```python
from build123d import *

# Parameters (mm, degrees)
BOSS_EXTRUDE1_DEPTH     = 55
CUT_EXTRUDE2_DEPTH      = 206.91260282
CUT_EXTRUDE2_DEPTH_BACK = 206.91260282
SKETCH2_W               = 100.4
SKETCH2_H               = 20.4
CUT_EXTRUDE3_DEPTH      = 20
FILLET1_R               = 45
CUT_EXTRUDE4_DEPTH      = 206.91260282
CUT_EXTRUDE4_DEPTH_BACK = 206.91260282
BOSS_EXTRUDE2_DEPTH     = 55
SKETCH29_R              = 1.75
SKETCH29_R_2            = 13
CUT_EXTRUDE5_DEPTH      = 10
SKETCH33_R              = 2.3
CUT_EXTRUDE9_DEPTH      = 10
SKETCH34_R              = 2.3
CUT_EXTRUDE10_DEPTH     = 10
FILLET2_R               = 5
CUT_EXTRUDE6_DEPTH      = 5
FILLET3_START           = 72
FILLET3_DEPTH           = 42
FILLET3_START_2         = 73.456949031
FILLET3_2_DEPTH         = 10
FILLET3_START_3         = 108.456949031
FILLET3_3_DEPTH         = 5
SKETCH31_R              = 2.3
CUT_EXTRUDE7_DEPTH      = 10
SKETCH32_R              = 2.3
CUT_EXTRUDE8_DEPTH      = 10
SKETCH35_R              = 2.3
CUT_EXTRUDE11_DEPTH     = 157.645539016
SKETCH36_R              = 4
CUT_EXTRUDE12_DEPTH     = 161.275509096
SKETCH37_R              = 2.1
CUT_EXTRUDE13_DEPTH     = 15
SKETCH38_R              = 2.3
CUT_EXTRUDE14_DEPTH     = 202.494416813
SKETCH39_R              = 4
CUT_EXTRUDE15_DEPTH     = 31
CHAMFER1_SIZE           = 1


with BuildPart() as part:
    # Sketch1 → Boss-Extrude1 (new body)
    with BuildSketch(Plane(origin=(0, 0, 0), x_dir=(1, 0, 0), z_dir=(0, 1, 0))):
        Polygon((0, 0), (150, 0), (75, 129.903810568), align=None)
    extrude(amount=-BOSS_EXTRUDE1_DEPTH)

    # Sketch4 → Cut-Extrude2 (cut, two sides: drawn at the far end of the back side and taken through both)
    with BuildSketch(Plane(origin=(0, 0, 0), x_dir=(1, 0, 0), z_dir=(0, 1, 0)).offset(-CUT_EXTRUDE2_DEPTH_BACK)):
        Polygon((58.511973189, 45.566570047), (40.845863577, 35.365169595), (51.047264029, 17.699059984), (68.713373641, 27.900460435), align=None)
    extrude(amount=CUT_EXTRUDE2_DEPTH + CUT_EXTRUDE2_DEPTH_BACK, mode=Mode.SUBTRACT)

    # Sketch2 → Cut-Extrude3 (cut)
    with BuildSketch(Plane(origin=(0, 0, 0), x_dir=(1, 0, 0), z_dir=(0, 1, 0))):
        Polygon((109.197045256, 138.33483042), (58.997045256, 51.38587988), (41.330127019, 61.58587988), (91.530127019, 148.53483042), align=None)
        with Locations((124.2, 15.2)):
            Rectangle(SKETCH2_W, SKETCH2_H)
    extrude(amount=-CUT_EXTRUDE3_DEPTH, mode=Mode.SUBTRACT)

    # Fillet1
    fillet1_edges = [part.edges().sort_by_distance(p)[0] for p in [
        (0, -27.5, 0),
    ]]
    fillet(fillet1_edges, radius=FILLET1_R)

    # Sketch27 → Cut-Extrude4 (cut, two sides: drawn at the far end of the back side and taken through both)
    with BuildSketch(Plane(origin=(0, 0, 0), x_dir=(1, 0, 0), z_dir=(0, 1, 0)).offset(-CUT_EXTRUDE4_DEPTH_BACK)):
        Polygon((238.272822489, 351.900634614), (92.551448183, 99.503810568), (65.734741667, 53.05591239), (78.81753352, 30.4), (132.448551817, 30.4), (423.891300428, 30.4), (928.68494852, 321.842748611), (743.066470581, 643.343383225), align=None)
    extrude(amount=CUT_EXTRUDE4_DEPTH + CUT_EXTRUDE4_DEPTH_BACK, mode=Mode.SUBTRACT)

    # Sketch28 → Boss-Extrude2 (add)
    with BuildSketch(Plane(origin=(0, 0, 0), x_dir=(1, 0, 0), z_dir=(0, 1, 0))):
        Polygon((83.054457118, 83.054539524), (113.460135283, 30.4), (107.686368323, 30.4), (80.167837876, 78.054768335), align=None)
    extrude(amount=-BOSS_EXTRUDE2_DEPTH)

    # Sketch29 → Cut-Extrude5 (cut)
    with BuildSketch(Plane(origin=(98.252102834, 0, -56.73626329), x_dir=(-0.5000686496051991, 0, -0.8659857652883405), z_dir=(0.8659857652883404, 0, -0.500068649605199))):
        with Locations((-15.510385308, -12)):
            Circle(SKETCH29_R)
        with Locations((15.489614692, -12)):
            Circle(SKETCH29_R)
        with Locations((15.489614692, -43)):
            Circle(SKETCH29_R)
        with Locations((-15.510385308, -43)):
            Circle(SKETCH29_R)
        with Locations((-0.010385308, -27.5)):
            Circle(SKETCH29_R_2)
    extrude(amount=-CUT_EXTRUDE5_DEPTH, mode=Mode.SUBTRACT)

    # Sketch33 → Cut-Extrude9 (cut)
    with BuildSketch(Plane(origin=(26.327172275, 0, 15.2), x_dir=(0.4999999999999997, 0, -0.8660254037844388), z_dir=(0.8660254037844389, 0, 0.49999999999999983))):
        with Locations((122.448551817, -10)):
            Circle(SKETCH33_R)
    extrude(amount=-CUT_EXTRUDE9_DEPTH, mode=Mode.SUBTRACT)

    # Sketch34 → Cut-Extrude10 (cut)
    with BuildSketch(Plane(origin=(0, 0, -30.4), x_dir=(-1, 0, 0), z_dir=(0, 0, -1))):
        with Locations((-122.448551817, -10)):
            Circle(SKETCH34_R)
    extrude(amount=-CUT_EXTRUDE10_DEPTH, mode=Mode.SUBTRACT)

    # Fillet2
    fillet2_edges = [part.edges().sort_by_distance(p)[0] for p in [
        (107.686368323, -27.5, -30.4),
        (113.460135283, -27.5, -30.4),
        (83.054457118, -27.5, -83.054539524),
        (80.167837876, -27.5, -78.054768335),
        (65.734741667, -27.5, -53.05591239),
        (78.81753352, -27.5, -30.4),
    ]]
    fillet(fillet2_edges, radius=FILLET2_R)

    # Sketch30 → Cut-Extrude6 (cut)
    with BuildSketch(Plane.XZ.offset(55)):
        Polygon((62.116998953, -39.323625207), (122.736002524, -74.32843068), (125.736414421, -69.132516088), (65.117410851, -34.127710616), align=None)
    extrude(amount=-CUT_EXTRUDE6_DEPTH, mode=Mode.SUBTRACT)

    # Fillet3: read off the stored shape, not the designer's step
    # Fillet3 outline → Fillet3 (cut)
    with BuildSketch(Plane(origin=(0, 0, 0), x_dir=(0.5000686496051991, 0, 0.8659857652883406), z_dir=(0.8659857652883404, 0, -0.5000686496051993)).offset(FILLET3_START)):
        with BuildLine():
            Line((-2.990935885, 55), (-5.490935885, 55))
            ThreePointArc((-5.490935885, 55), (-3.723168932, 54.267766953), (-2.990935885, 52.5))
            Line((-2.990935885, 52.5), (-2.990935885, 55))
        make_face()
        with BuildLine():
            Line((5.509064115, 55), (3.009064115, 55))
            Line((3.009064115, 55), (3.009064115, 52.5))
            ThreePointArc((3.009064115, 52.5), (3.741297162, 54.267766953), (5.509064115, 55))
        make_face()
    extrude(amount=FILLET3_DEPTH, mode=Mode.SUBTRACT)

    # Fillet3 2 outline → Fillet3 2 (add)
    with BuildSketch(Plane(origin=(0, 0, 0), x_dir=(0.5000686496051991, 0, 0.8659857652883406), z_dir=(0.8659857652883404, 0, -0.5000686496051993)).offset(FILLET3_START_2)):
        with BuildLine():
            ThreePointArc((-0.490935885, 50), (-2.258702838, 50.732233047), (-2.990935885, 52.5))
            Line((-2.990935885, 52.5), (-2.990935885, 50))
            Line((-2.990935885, 50), (-0.490935885, 50))
        make_face()
        with BuildLine():
            ThreePointArc((3.009064115, 52.5), (2.276831068, 50.732233047), (0.509064115, 50))
            Line((0.509064115, 50), (3.009064115, 50))
            Line((3.009064115, 50), (3.009064115, 52.5))
        make_face()
    extrude(amount=FILLET3_2_DEPTH)

    # Fillet3 3 outline → Fillet3 3 (add)
    with BuildSketch(Plane(origin=(0, 0, 0), x_dir=(0.5000686496051991, 0, 0.8659857652883406), z_dir=(0.8659857652883404, 0, -0.5000686496051993)).offset(FILLET3_START_3)):
        with BuildLine():
            ThreePointArc((-0.490935885, 50), (-2.258702838, 50.732233047), (-2.990935885, 52.5))
            Line((-2.990935885, 52.5), (-2.990935885, 50))
            Line((-2.990935885, 50), (-0.490935885, 50))
        make_face()
        with BuildLine():
            ThreePointArc((3.009064115, 52.5), (2.276831068, 50.732233047), (0.509064115, 50))
            Line((0.509064115, 50), (3.009064115, 50))
            Line((3.009064115, 50), (3.009064115, 52.5))
        make_face()
    extrude(amount=FILLET3_3_DEPTH)

    # Sketch31 → Cut-Extrude7 (cut)
    with BuildSketch(Plane(origin=(4.330127019, 0, 2.5), x_dir=(0.5000000000000019, 0, -0.8660254037844376), z_dir=(0.8660254037844376, 0, 0.5000000000000019))):
        with Locations((89, -10)):
            Circle(SKETCH31_R)
        with Locations((132.113248654, -10)):
            Circle(SKETCH31_R)
    extrude(amount=-CUT_EXTRUDE7_DEPTH, mode=Mode.SUBTRACT)

    # Sketch32 → Cut-Extrude8 (cut)
    with BuildSketch(Plane(origin=(0, 0, -5), x_dir=(-1, 0, 0), z_dir=(0, 0, -1))):
        with Locations((-132.113248654, -10)):
            Circle(SKETCH32_R)
        with Locations((-89, -10)):
            Circle(SKETCH32_R)
    extrude(amount=-CUT_EXTRUDE8_DEPTH, mode=Mode.SUBTRACT)

    # Sketch35 → Cut-Extrude11 (cut, through all)
    with BuildSketch(Plane(origin=(45.946562611, 0, -26.532116854), x_dir=(-0.5000686496051995, 0, -0.8659857652883403), z_dir=(0.8659857652883401, 0, -0.5000686496051994))):
        with Locations((0, -15)):
            Circle(SKETCH35_R)
        with Locations((0, -40)):
            Circle(SKETCH35_R)
    extrude(amount=-CUT_EXTRUDE11_DEPTH, mode=Mode.SUBTRACT)

    # Sketch36 → Cut-Extrude12 (cut, through all)
    with BuildSketch(Plane(origin=(42.482619549, 0, -24.531842256), x_dir=(-0.5000686496051995, 0, -0.8659857652883403), z_dir=(0.8659857652883401, 0, -0.5000686496051994))):
        with Locations((0, -15)):
            Circle(SKETCH36_R)
        with Locations((0, -40)):
            Circle(SKETCH36_R)
    extrude(amount=-CUT_EXTRUDE12_DEPTH, mode=Mode.SUBTRACT)

    # Sketch37 → Cut-Extrude13 (cut)
    with BuildSketch(Plane.XZ.offset(55)):
        with Locations(Location((69.166562249, -15.2, 0), (0, 0, 270))):
            Circle(SKETCH37_R)
        with Locations(Location((105.195419079, -15.2, 0), (0, 0, 270))):
            Circle(SKETCH37_R)
        with Locations(Location((47.746867262, -52.3, 0), (0, 0, 270))):
            Circle(SKETCH37_R)
        with Locations(Location((65.761295677, -83.501905284, 0), (0, 0, 270))):
            Circle(SKETCH37_R)
    extrude(amount=-CUT_EXTRUDE13_DEPTH, mode=Mode.SUBTRACT)

    # Sketch38 → Cut-Extrude14 (cut, through all)
    with BuildSketch(Plane(origin=(0, -20, 0), x_dir=(1, 0, 0), z_dir=(0, 1, 0))):
        with Locations(Location((89, 15.2, 0), (0, 0, 270))):
            Circle(SKETCH38_R)
        with Locations(Location((126.224275908, 15.2, 0), (0, 0, 270))):
            Circle(SKETCH38_R)
        with Locations(Location((76.275724092, 101.713429511, 0), (0, 0, 270))):
            Circle(SKETCH38_R)
        with Locations(Location((57.663586138, 69.476260937, 0), (0, 0, 270))):
            Circle(SKETCH38_R)
    extrude(amount=-CUT_EXTRUDE14_DEPTH, mode=Mode.SUBTRACT)

    # Sketch39 → Cut-Extrude15 (cut)
    with BuildSketch(Plane.XZ.offset(55)):
        with Locations(Location((89, -15.2, 0), (0, 0, 270))):
            Circle(SKETCH39_R)
        with Locations(Location((126.224275908, -15.2, 0), (0, 0, 270))):
            Circle(SKETCH39_R)
        with Locations(Location((57.663586138, -69.476260937, 0), (0, 0, 270))):
            Circle(SKETCH39_R)
        with Locations(Location((76.275724092, -101.713429511, 0), (0, 0, 270))):
            Circle(SKETCH39_R)
    extrude(amount=-CUT_EXTRUDE15_DEPTH, mode=Mode.SUBTRACT)

    # Chamfer1
    chamfer1_edges = [part.edges().sort_by_distance(p)[0] for p in [
        (105.195419079, -55, -13.1),
        (69.166562249, -55, -13.1),
        (47.746867262, -55, -50.2),
        (65.761295677, -55, -81.401905284),
    ]]
    chamfer(chamfer1_edges, length=CHAMFER1_SIZE)


solid = part.part
```
Geometry check sheet. Reference: the model listing, model coordinates, mm. A direction names the side the tool comes from. Coordinates: 2 decimals unless noted, no trailing zeros. Order: outer loops, then holes, each group sorted by start corner. A loop starts at its lowest first (then second) coordinate and runs counter-clockwise, first axis right, second up. Notation, with made-up numbers: (-12, 73) - (39, 73) arc R12 ccw to (39, 80) - close; hole circle Ø11 at (53, 34). An arc over 180 degrees is marked (long way). Answer in a Markdown table with one row per item. Add a question column.
1. Section check D-D (x = 141.5). Enter the section's corners in (y, z).
2. Access from +Z, -Z, +X, -X, +Y, -Y to the whole of each face (thin tool, end or side, straight path). Record for faces 3 (the face through (55.9, -24, -71.2)), 4 (the face through (41.18, -39.94, -26.79)), 5 (the face through (90, -28, -30.4)), 6 (the face through (91.298, -9.899, -2.535)).
3. Gauge pin test, flat ends, axial feed: pin 1 Ø5 at (x, y) = (125, -20) entering from -Z; pin 2 Ø3 at (x, z) = (76.28, -101.71) entering from +Y; pin 3 Ø3 at (x, z) = (69.5, -40.5) entering from -Y; pin 4 Ø3.5 at (x, y) = (122.45, -10) entering from -Z. Record the tip position at first contact, or that the pin passes through.
4. Section check A-A (y = -4). Give the number of separate pieces and of enclosed holes in the cut face, plus the area to 3 significant figures.
5. Material ranges on L1, parallel to X at y = -14, z = -32; L2, parallel to X at y = -43.75, z = -15.2; L3, parallel to X at y = -11.5, z = -70, recorded low to high. Write a range as [from, to].
6. Draft check along X on faces 1 (the face through (128.505, -21.972, -15.499)), 2 (the face through (73.7, -24, -101.7)). Enter one of: +X half, -X half, draft (parallel to the pull), parting line (faces both ways), or undercut.
Data:
| question | item | result |
|---|---|---|
| 1 | outline | (-55, -14.72) - (-20, -14.72) - (-20, -5) - (0, -5) - (0, 0) - (-55, 0) - close |
| 2 | face 3 | -Y |
| 2 | face 4 | none |
| 2 | face 5 | +Y, -Y |
| 2 | face 6 | +Z |
| 3 | pin 1 | stops at z = -30.4 |
| 3 | pin 2 | passes through |
| 3 | pin 3 | stops at y = -50.38 |
| 3 | pin 4 | stops at z = -5 |
| 4 | separate pieces | 1 |
| 4 | enclosed holes | 2 |
| 4 | area | 3,070 mm² |
| 5 | L1 | x = [34.86, 42.79], [66.35, 78.04], [102.69, 112.68] |
| 5 | L2 | x = [44.22, 67.07], [71.27, 85], [93, 103.1], [107.3, 122.22], [130.22, 141.22] |
| 5 | L3 | x = [40.41, 46.19], [69.74, 75.52], [84.82, 86.89] |
| 6 | face 1 | undercut |
| 6 | face 2 | undercut |
